Part model, mm, in its own coordinate system. A direction names the side the tool comes from. Round coordinates to 2 decimals unless told otherwise and drop trailing zeros. Order: outer loops, then holes, each group sorted by start corner. A loop starts at its lowest first (then second) coordinate and runs counter-clockwise, first axis right, second up. Notation, with made-up numbers: (31.25, 16.25) -> (71.25, 16.25) arc R27 cw to (71.25, 41.25) -> close; hole circle Ø3 at (-14, 81.25). An arc over 180 degrees is marked (long way). Answer as a JSON object with one key per item and string values. Group by question number.
```python
from build123d import *

# Parameters (mm, degrees)
SKETCH3_W            = 20
SKETCH3_H            = 50
BOSS_EXTRUDE3_DEPTH  = 5
CUT_EXTRUDE2_DEPTH   = 2
SKETCH6_R            = 3.57
CUT_EXTRUDE3_DEPTH   = 3
SKETCH8_W            = 1.25
SKETCH8_H            = 50
CUT_EXTRUDE5_DEPTH   = 30
SKETCH9_W            = 70
SKETCH9_H            = 20
BOSS_EXTRUDE4_DEPTH  = 20
SKETCH10_W           = 70
SKETCH10_H           = 10
CUT_EXTRUDE6_DEPTH   = 10
SKETCH11_W           = 30
SKETCH11_H           = 10
BOSS_EXTRUDE5_DEPTH  = 25
SKETCH12_W           = 20
SKETCH12_H           = 1.5
CUT_EXTRUDE7_DEPTH   = 1
SKETCH13_W           = 15
SKETCH13_H           = 38.806898948
CUT_EXTRUDE8_DEPTH   = 13
BOSS_EXTRUDE6_DEPTH  = 2
SKETCH16_R           = 0.75
CUT_EXTRUDE9_DEPTH   = 0.5
SKETCH19_W           = 70
SKETCH19_H           = 10
BOSS_EXTRUDE8_DEPTH  = 10
BOSS_EXTRUDE9_DEPTH  = 2
FILLET1_R            = 6
FILLET2_R            = 4
SKETCH22_W           = 15
SKETCH22_H           = 5
BOSS_EXTRUDE10_DEPTH = 25
FILLET3_R            = 5


with BuildPart() as part:
    # Sketch3 → Boss-Extrude3 (new body)
    with BuildSketch(Plane.XY):
        Rectangle(SKETCH3_W, SKETCH3_H)
    extrude(amount=BOSS_EXTRUDE3_DEPTH)

    # Sketch4 → Cut-Extrude2 (cut)
    with BuildSketch(Plane.XY.offset(5)):
        with BuildLine():
            Line((-2.85, 14.850023256), (-1.8, 2.795667197))
            Line((-1.8, 2.795667197), (1.8, 2.795667197))
            Line((1.8, 2.795667197), (2.85, 14.850023256))
            ThreePointArc((2.85, 14.850023256), (0, 13.43), (-2.85, 14.850023256))
        make_face()
        with BuildLine():
            Line((1.8, 2.795667197), (-1.8, 2.795667197))
            ThreePointArc((-1.8, 2.795667197), (0, 0.995667197), (1.8, 2.795667197))
        make_face()
        with BuildLine():
            ThreePointArc((3.57, 17), (-1.133666618, 20.385217866), (-2.85, 14.850023256))
            Line((-2.85, 14.850023256), (2.85, 14.850023256))
            ThreePointArc((2.85, 14.850023256), (3.385217866, 15.866333382), (3.57, 17))
        make_face()
        with BuildLine():
            Line((2.85, 14.850023256), (-2.85, 14.850023256))
            ThreePointArc((-2.85, 14.850023256), (0, 13.43), (2.85, 14.850023256))
        make_face()
    extrude(amount=-CUT_EXTRUDE2_DEPTH, mode=Mode.SUBTRACT)

    # Sketch6 → Cut-Extrude3 (cut)
    with BuildSketch(Plane.XY.offset(3)):
        with Locations((0, 17)):
            Circle(SKETCH6_R)
    extrude(amount=-CUT_EXTRUDE3_DEPTH, mode=Mode.SUBTRACT)

    # Sketch8 → Cut-Extrude5 (cut)
    with BuildSketch(Plane(origin=(10, 0, 0), x_dir=(0, 0, -1), z_dir=(1, 0, 0))):
        with Locations((-0.625, 0)):
            Rectangle(SKETCH8_W, SKETCH8_H)
    extrude(amount=-CUT_EXTRUDE5_DEPTH, mode=Mode.SUBTRACT)

    # Sketch9 → Boss-Extrude4 (add)
    with BuildSketch(Plane.XY.offset(5)):
        with Locations((0, -15)):
            Rectangle(SKETCH9_W, SKETCH9_H)
    extrude(amount=BOSS_EXTRUDE4_DEPTH)

    # Sketch10 → Cut-Extrude6 (cut)
    with BuildSketch(Plane.XY.offset(25)):
        with Locations((0, -20)):
            Rectangle(SKETCH10_W, SKETCH10_H)
    extrude(amount=-CUT_EXTRUDE6_DEPTH, mode=Mode.SUBTRACT)

    # Sketch11 → Boss-Extrude5 (add)
    with BuildSketch(Plane(origin=(0, -25, 0), x_dir=(-1, 0, 0), z_dir=(0, -1, 0))):
        with Locations((0, -10)):
            Rectangle(SKETCH11_W, SKETCH11_H)
    extrude(amount=BOSS_EXTRUDE5_DEPTH)

    # Sketch12 → Cut-Extrude7 (cut)
    with BuildSketch(Plane.XY.offset(15)):
        with Locations((0, -15.75)):
            Rectangle(SKETCH12_W, SKETCH12_H)
    extrude(amount=-CUT_EXTRUDE7_DEPTH, mode=Mode.SUBTRACT)

    # Sketch13 → Cut-Extrude8 (cut)
    with BuildSketch(Plane(origin=(0, -5, 0), x_dir=(1, 0, 0), z_dir=(0, 1, 0))):
        with Locations((0, 1.403449474)):
            Rectangle(SKETCH13_W, SKETCH13_H)
    extrude(amount=-CUT_EXTRUDE8_DEPTH, mode=Mode.SUBTRACT)

    # Sketch15 → Boss-Extrude6 (add)
    with BuildSketch(Plane.XZ.offset(50)):
        with BuildLine():
            Line((0, 7.1), (5.553473382, 11.361330003))
            ThreePointArc((5.553473382, 11.361330003), (0, 14.1), (-5.553473382, 11.361330003))
            Line((-5.553473382, 11.361330003), (0, 7.1))
        make_face()
    extrude(amount=BOSS_EXTRUDE6_DEPTH)

    # Sketch16 → Cut-Extrude9 (cut)
    with BuildSketch(Plane(origin=(0, -52, 0), x_dir=(-1, 0, 0), z_dir=(0, -1, 0))):
        with Locations((-1.5, -11.498525774)):
            Circle(SKETCH16_R)
        with Locations((1.5, -11.498525774)):
            Circle(SKETCH16_R)
    extrude(amount=-CUT_EXTRUDE9_DEPTH, mode=Mode.SUBTRACT)

    # Sketch19 → Boss-Extrude8 (add)
    with BuildSketch(Plane.XY.offset(25)):
        with Locations((0, -10)):
            Rectangle(SKETCH19_W, SKETCH19_H)
    extrude(amount=BOSS_EXTRUDE8_DEPTH)

    # Sketch21 → Boss-Extrude9 (add)
    with BuildSketch(Plane(origin=(0, -11, 0), x_dir=(-1, 0, 0), z_dir=(0, -1, 0))):
        with BuildLine():
            Line((-24.95459775, -30.351053915), (-33.467453748, -26.18260363))
            add(Edge.make_bspline(
                [(-33.467453748, -26.18260363), (-45.809189014, -35.587529887), (-43.975470741, -50.179256657)],
                knots=[0, 0, 0, 1, 1, 1], degree=2))
            add(Edge.make_bspline(
                [(-24.95459775, -30.351053915), (-30.210326616, -44.560066847), (-43.975470741, -50.179256657)],
                knots=[0, 0, 0, 1, 1, 1], degree=2))
        make_face()
        with BuildLine():
            Line((24.95459775, -30.351053915), (33.467453748, -26.18260363))
            add(Edge.make_bspline(
                [(33.467453748, -26.18260363), (45.809189014, -35.587529887), (43.975470741, -50.179256657)],
                knots=[0, 0, 0, 1, 1, 1], degree=2))
            add(Edge.make_bspline(
                [(24.95459775, -30.351053915), (30.210326616, -44.560066847), (43.975470741, -50.179256657)],
                knots=[0, 0, 0, 1, 1, 1], degree=2))
        make_face()
    extrude(amount=-BOSS_EXTRUDE9_DEPTH)

    # Fillet1
    fillet1_edges = [part.edges().sort_by_distance(p)[0] for p in [
        (-15, -25, 10),
        (15, -25, 10),
    ]]
    fillet(fillet1_edges, radius=FILLET1_R)

    # Fillet2
    fillet2_edges = [part.edges().sort_by_distance(p)[0] for p in [
        (35, -25, 10),
        (-35, -25, 10),
        (-15, -50, 10),
        (15, -50, 10),
    ]]
    fillet(fillet2_edges, radius=FILLET2_R)

    # Sketch22 → Boss-Extrude10 (add)
    with BuildSketch(Plane(origin=(0, 0, 1.25), x_dir=(-1, 0, 0), z_dir=(0, 0, -1))):
        with Locations((0, -7.5)):
            Rectangle(SKETCH22_W, SKETCH22_H)
    extrude(amount=-BOSS_EXTRUDE10_DEPTH)

    # Fillet3
    fillet3_edges = [part.edges().sort_by_distance(p)[0] for p in [
        (0, -5, 5),
    ]]
    fillet(fillet3_edges, radius=FILLET3_R)


solid = part.part
```
Q1. Band-saw the part on B-B (y = -22.5). List the corners of the cut face in (x, z), plus the area to 3 significant figures.
Q2. Band-saw the part on A-A (y = 19.5). List the corners of the cut face in (x, z).
Q3. Which spindle directions (+Z, -Z, +X, -X, +Y, -Y) get a long thin tool onto all of the face, cutting with end or side? Do faces 1 (the flat face through (-15, -38, 10)), 2 (the flat face through (0, -52, 11)), 3 (the flat face through (-2.332, 8.907, 4.014)), 4 (the flat face through (0, -10, 10)). Say none if no direction does.
Q4. Wall check: line 1 (Y direction, x = 0, z = 4); line 2 (X direction, y = 17, z = 4.25); line 3 (Y direction, x = -1.5, z = 21). Give the ranges that are in metal, low to high. Write a range as [from, to].
Q5. Band-saw the part on C-C (z = 25). List the corners of the cut face in (x, y), plus the area to 3 significant figures.
Q6. Band-saw the part on D-D (x = -17). List the corners of the cut face in (y, z), plus the area to 3 significant figures.
Q7. Two-plate mould, pull along X, no slides. Class faces 5 (the cylindrical face through (0.1, -51, 14.1)), 6 (the flat face through (36, -9, 39)), 7 (the flat face through (0, 8, 3)): +X half, -X half, draft (parallel to the pull), parting line (faces both ways), or undercut.
Q8. Drop flat-ended pins along their axis: pin 1 Ø3 at (x, y) = (18, -33.5) entering from -Z; pin 2 Ø0.8 at (x, z) = (-9.5, 14.5) entering from +Y; pin 3 Ø3 at (y, z) = (-37.5, 10) entering from +X; pin 4 Ø8.5 at (x, z) = (-35, 43) entering from +Y. Give the stop position or say it passes through.
Completed:
{
 "1": {"outline": "(-34.71, 5) -> (-10, 5) -> (-10, 1.25) -> (10, 1.25) -> (10, 5) -> (34.71, 5) -> (34.71, 15) -> (-34.71, 15) -> close", "area": "769 mm2"},
 "2": {"outline": "(-10, 1.25) -> (-2.55, 1.25) -> (-2.55, 5) -> (-10, 5) -> close; (2.55, 1.25) -> (10, 1.25) -> (10, 5) -> (2.55, 5) -> close"},
 "3": {"face 1": "+Z, -Z, -X, -Y", "face 2": "+Z, -Z, +X, -X, -Y", "face 3": "+Z", "face 4": "-Z"},
 "4": {"line 1": "[-25, -18], [-10, 1], [20.57, 25]", "line 2": "[-10, -3.57], [3.57, 10]", "line 3": "[-15, -5]"},
 "5": {"outline": "(-35, -15) -> (35, -15) -> (35, -5) -> (-35, -5) -> close", "area": "700 mm2"},
 "6": {"outline": "(-26.53, 5) -> (-5, 5) -> (-5, 35) -> (-15, 35) -> (-15, 15) -> (-26.53, 15) -> close", "area": "415 mm2"},
 "7": {"face 5": "parting line", "face 6": "draft", "face 7": "undercut"},
 "8": {"pin 1": "through", "pin 2": "y = -5", "pin 3": "x = 15", "pin 4": "y = -9"}
}
